Build history of the part. All positions in model axes, mm. A direction names the side the tool comes from. Give positions to 0.01 mm unless a question says otherwise; leave off trailing zeros. Write each loop counter-clockwise with the first axis right and the second up, starting at its lowest first coordinate (ties: lowest second). Pieces come first, ordered by that corner, then holes.
from build123d import *

# Parameters (mm, degrees)
F0_R      = 4.2
F0_R_2    = 2.9
F0_R_3    = 1.5
F1_DEPTH  = 1.5
F2_DEPTH  = 5
F3_DEPTH  = 3
F5_DEPTH  = 4.5
F7_W      = 1
F7_H      = 5
F8_DEPTH  = 10
F9_R      = 1
F10_DEPTH = 2
F11_R     = 1
F12_W     = 2.2280928679
F12_H     = 1.1955168769
F13_DEPTH = 3


with BuildPart() as f1:
    # F0 (on Top) → F1 (new body)
    with BuildSketch(Plane.XY):
        with BuildLine():
            Line((1.3210678119, -5.75), (5.5433312065, -1.5277366054))
            ThreePointArc((5.5433312065, -1.5277366054), (4.0658639918, 4.0658639918), (-1.5277366054, 5.5433312065))
            Line((-1.5277366054, 5.5433312065), (-5.75, 1.3210678119))
            Line((-5.75, 1.3210678119), (-5.75, 0))
            ThreePointArc((-5.75, 0), (-4.0658639918, -4.0658639918), (0, -5.75))
            Line((0, -5.75), (1.3210678119, -5.75))
        make_face()
        Circle(F0_R, mode=Mode.SUBTRACT)
        with BuildLine():
            ThreePointArc((-1.5277366054, 5.5433312065), (4.0658639918, 4.0658639918), (5.5433312065, -1.5277366054))
            Line((5.5433312065, -1.5277366054), (1.3210678119, -5.75))
            Line((1.3210678119, -5.75), (20, -5.75))
            Line((20, -5.75), (20, 0.75))
            Line((20, 0.75), (0.75, 20))
            Line((0.75, 20), (-5.75, 20))
            Line((-5.75, 20), (-5.75, 1.3210678119))
            Line((-5.75, 1.3210678119), (-1.5277366054, 5.5433312065))
        make_face()
        Circle(F0_R)
        Circle(F0_R_2, mode=Mode.SUBTRACT)
        Circle(F0_R_2)
        Circle(F0_R_3, mode=Mode.SUBTRACT)
    extrude(amount=F1_DEPTH)

    # F0 (on Top) → F2 (join)
    with BuildSketch(Plane.XY):
        with BuildLine():
            Line((1.3210678119, -5.75), (5.5433312065, -1.5277366054))
            ThreePointArc((5.5433312065, -1.5277366054), (4.0658639918, 4.0658639918), (-1.5277366054, 5.5433312065))
            Line((-1.5277366054, 5.5433312065), (-5.75, 1.3210678119))
            Line((-5.75, 1.3210678119), (-5.75, 0))
            ThreePointArc((-5.75, 0), (-4.0658639918, -4.0658639918), (0, -5.75))
            Line((0, -5.75), (1.3210678119, -5.75))
        make_face()
        Circle(F0_R, mode=Mode.SUBTRACT)
    extrude(amount=-F2_DEPTH)

    # F0 (on Top) → F3 (join)
    with BuildSketch(Plane.XY):
        Circle(F0_R_2)
        Circle(F0_R_3, mode=Mode.SUBTRACT)
    extrude(amount=-F3_DEPTH)

    # F4 (on Top) → F5 (join)
    with BuildSketch(Plane.XY):
        with BuildLine():
            ThreePointArc((0, -5.75), (-4.0658639918, -4.0658639918), (-5.75, 0))
            Line((-5.75, 0), (-5.75, 20))
            Line((-5.75, 20), (-7.25, 20))
            Line((-7.25, 20), (-7.25, 0))
            ThreePointArc((-7.25, 0), (-5.1265241636, -5.1265241636), (0, -7.25))
            Line((0, -7.25), (20, -7.25))
            Line((20, -7.25), (20, -5.75))
            Line((20, -5.75), (0, -5.75))
        make_face()
    extrude(amount=F5_DEPTH)

    # F7 (on offset) → F8 (cut)
    with BuildSketch(Plane(origin=(-3.5355339059, 3.5355339059, 0), x_dir=(-0.7071067812, -0.7071067812, 0), z_dir=(-0.7071067812, 0.7071067812, 0))):
        with Locations((-5.2581984438, -2.5)):
            Rectangle(F7_W, F7_H)
    extrude(amount=-F8_DEPTH, mode=Mode.SUBTRACT)

    # F9 (on face) → F10 (join)
    with BuildSketch(Plane(origin=(3.3645543858, 3.3645543858, 0), x_dir=(-0.7071067812, 0.7071067812, 0), z_dir=(0.7071067812, 0.7071067812, 0))):
        with Locations((0, -3.1)):
            Circle(F9_R)
    extrude(amount=F10_DEPTH)

    # F11
    f11_edges = [f1.edges().sort_by_distance(p)[0] for p in [
        (5.485875, 4.071661, -3.1),
    ]]
    fillet(f11_edges, radius=F11_R)

    # F12 (on face) → F13 (cut)
    with BuildSketch(Plane(origin=(3.3645543858, 3.3645543858, 0), x_dir=(-0.7071067812, 0.7071067812, 0), z_dir=(0.7071067812, 0.7071067812, 0))):
        with Locations((-0.035953708, -2.5022415616)):
            Rectangle(F12_W, F12_H)
    extrude(amount=F13_DEPTH, mode=Mode.SUBTRACT)


solid = f1.part
1. Saw through at B-B on z = -3.5. Give the cut face in (x, y), plus the area to 3 significant figures.
2. Drill centre lines: line 1 along Y through (x, z) = (0, -1.85); line 2 along Y through (x, z) = (0, -3.7); line 3 along Z through (x, y) = (1.25, 7.5). Where is each one in solid material? Low to high.
3. Drop flat-ended pins along their axis: pin 1 (1 mm diameter, centred on x = 2, z = -1.5, fed in from -Y); pin 2 (11 mm diameter, centred on x = 0, y = 0, fed in from -Z); pin 3 (3 mm diameter, centred on x = 15.5, y = 2.5, fed in from +Z); pin 4 (1.5 mm diameter, centred on y = 6.5, z = 3, fed in from +X). Give the stop position or say it passes through.
4. Saw through at A-A on z = -1. Give the cut face in (x, y).
5. Saw through at C-C on x = 15.25. Give the cut face in (y, z), plus the area to 3 significant figures.
6. 3-axis set-ups, long thin cutter, end or side, ignore diameter. For faces 4 (the face through (1.2, -1.2, -3)), 5 (the face through (3.4, -3.67, -2.46)), 6 (the face through (5.745, -0.247, -2.465)), 7 (the face through (4, 4, 1.5)), 8 (the face through (1, -5.75, -2)): which of +Z, -Z, +X, -X, +Y, -Y reach the whole face in a straight line?
7. Saw through at D-D on y = 9.25. Give the cut face in (x, z), plus the area to 3 significant figures.
8. Mould opens along Z. For faces 1 (the face through (-1, -3, 0)), 2 (the face through (-5.75, 1, -3)), 3 (the face through (4, 4, -3.1)) say: pulls with the +Z half, pulls with the -Z half, needs draft (parallel to the pull), parting line crosses it, or undercut.
Outcome:
1. outline: (-5.75, 0) arc R5.75 ccw to (0, -5.75) - (1.32, -5.75) - (5.54, -1.53) arc R5.75 ccw to (5.65, 1.08) - (4.01, 2.72) - (4.72, 3.42) arc R0.92 ccw to (3.42, 4.72) - (2.72, 4.01) - (1.08, 5.65) arc R5.75 ccw to (-1.53, 5.54) - (-5.75, 1.32) - close; hole circle Ø8.4 at (0, 0)
1. area: 41.7 mm2
2. line 1: y = -5.75 to -4.2, -2.9 to -1.5, 1.5 to 2.9, 4.2 to 5.75
2. line 2: y = -5.75 to -4.2, 4.2 to 5.75
2. line 3: z = 0 to 1.5
3. pin 1: stops at y = -5.57
3. pin 2: stops at z = -5
3. pin 3: stops at z = 1.5
3. pin 4: stops at x = -5.75
4. outline: (-5.75, 0) arc R5.75 ccw to (0, -5.75) - (1.32, -5.75) - (5.54, -1.53) arc R5.75 ccw to (5.65, 1.08) - (1.08, 5.65) arc R5.75 ccw to (-1.53, 5.54) - (-5.75, 1.32) - close; circle Ø5.8 at (0, 0); hole circle Ø8.4 at (0, 0); hole circle Ø3 at (0, 0)
5. outline: (-7.25, 0) - (5.5, 0) - (5.5, 1.5) - (-5.75, 1.5) - (-5.75, 4.5) - (-7.25, 4.5) - close
5. area: 23.6 mm2
6. face 4: -Z
6. face 5: -Z, +X, -Y
6. face 6: -Z, +X
6. face 7: +Z, +X, +Y
6. face 8: -Z, +X, -X, -Y
7. outline: (-7.25, 0) - (11.5, 0) - (11.5, 1.5) - (-5.75, 1.5) - (-5.75, 4.5) - (-7.25, 4.5) - close
7. area: 32.6 mm2
8. face 1: pulls with the -Z half
8. face 2: needs draft
8. face 3: undercut
